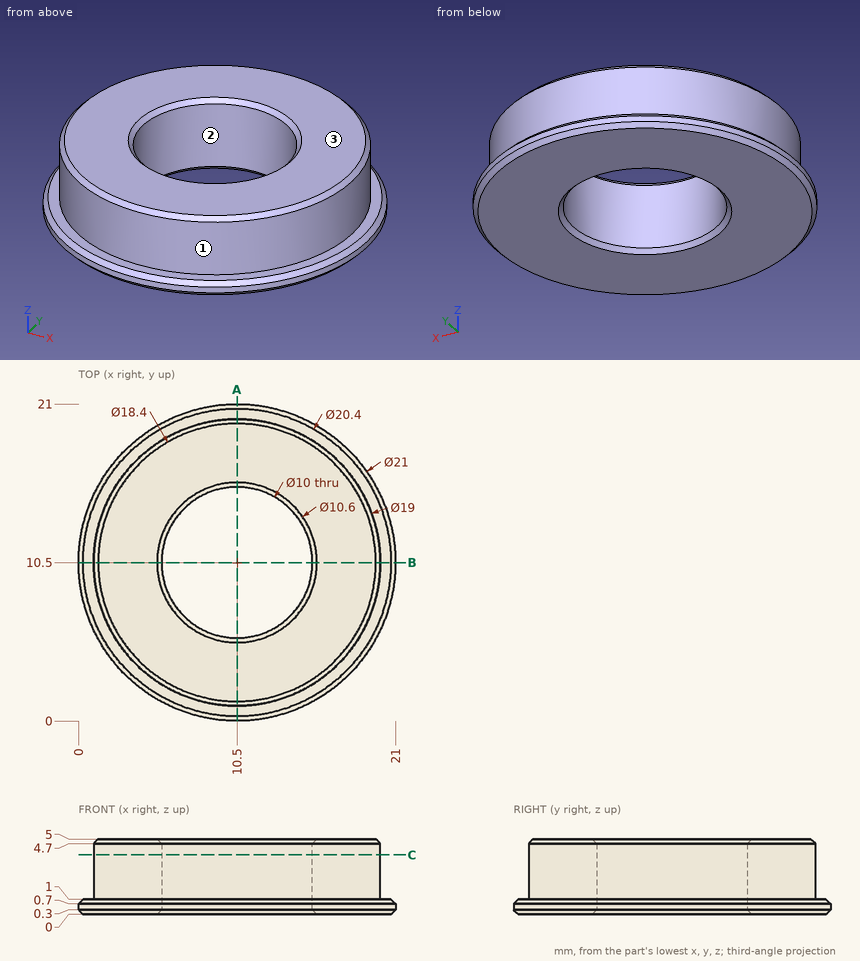
Answer from the drawing. Dimensions are ordinates in mm from the lowest x, y and z of the part. Round coordinates to 2 decimals unless told otherwise and drop trailing zeros. Order: outer loops, then holes, each group sorted by start corner. A loop starts at its lowest first (then second) coordinate and runs counter-clockwise, first axis right, second up.
1) The part is cut by section C-C on z = 3.95. Write down the section's boundary in (x, y), plus the area to 3 significant figures.
2) The mould has two halves that part along Y. Classify the marked faces 1, 2 and 3: released by +Y, released by -Y, zero draft, split by the parting line, or undercut.
3) Straight lines are drawn through the part: L1, parallel to Y at x = 10.5, z = 3.2; L2, parallel to X at y = 13.5, z = 1.45; L3, parallel to X at y = 12, z = 4.1. For each, find the intervals that lie inside material, in ascending order.
4) The part is cut by section A-A on x = 10.5. Write down the section's boundary in (y, z), plus the area to 4 significant figures.
5) Flat-ended cylindrical pins translate along their axes: pin 1 (2 mm diameter, centred on x = 12.5, z = 3, fed in from -Y); pin 2 (3 mm diameter, centred on x = 2.5, y = 18, fed in from +Z); pin 3 (1 mm diameter, centred on y = 2, z = 0.5, fed in from +X). Find the tip coordinate at first contact, or state that the pin passes through.
Resolved:
1. outline: circle Ø19 at (10.5, 10.5); hole circle Ø10 at (10.5, 10.5)
1. area: 205 mm2
2. face 1: split by the parting line
2. face 2: undercut
2. face 3: zero draft
3. L1: y = 1 to 5.5, 15.5 to 20
3. L2: x = 1.49 to 6.5, 14.5 to 19.51
3. L3: x = 1.12 to 5.73, 15.27 to 19.88
4. outline: (0, 0.3) - (0.3, 0) - (5.2, 0) - (5.5, 0.3) - (5.5, 4.7) - (5.2, 5) - (1.3, 5) - (1, 4.7) - (1, 1) - (0.3, 1) - (0, 0.7) - close; (15.5, 0.3) - (15.8, 0) - (20.7, 0) - (21, 0.3) - (21, 0.7) - (20.7, 1) - (20, 1) - (20, 4.7) - (19.7, 5) - (15.8, 5) - (15.5, 4.7) - close
4. area: 46.55 mm2
5. pin 1: stops at y = 1.05
5. pin 2: stops at z = 4.73
5. pin 3: stops at x = 17.3
